Geometry: final body of the model. Coordinates: model frame, mm. A direction names the side the tool comes from. Round coordinates to 2 decimals unless told otherwise and drop trailing zeros. Loops run counter-clockwise (first coordinate to the right, second up) from the corner with the lowest first, then second, coordinate; pieces in that order, holes last. Notation, with made-up numbers: (41.5, -12) - (48.5, -12) arc R12 cw to (48.5, 8) - close; hole circle Ø3 at (73, 69). An arc over 180 degrees is marked (long way). Return JSON: item names as keys, results as strings. Group by question number.
1. Section C-C on z = 2. Return loops of the section in (x, y).
2. Section A-A on x = 0. Return loops of the section in (y, z) (1 decimal).
3. Section D-D on y = -15.5. Count the separate pieces of the cut face and the enclosed holes in it, and give its area (3 significant figures).
4. Draft query along X for faces 1 (the face through (39, 0, 4)), 2 (the face through (67.6, -12.5, 4.3)). Return one class per face: +X half, -X half, draft (parallel to the pull), parting line (faces both ways), or undercut.
5. Set-up query: faces 3 (the face through (16, 0, 4.762)), 4 (the face through (-13, 25.4, 7)), 5 (the face through (-16, -13, -4.762)). Return all of +Z, -Z, +X, -X, +Y, -Y with unobstructed straight access to the full face (end or side cutting, diameter ignored); none if empty.
6. Material intervals for probe 1 along X at (y, z) = (-19, -12); probe 2 along Y at (x, z) = (67.5, -10); probe 3 along X at (y, z) = (-13, -2), sorted ascending.
7. First-contact query: pin 1 Ø1 at (x, y) = (1.5, -18.5) entering from -Z; pin 2 Ø1.7 at (x, y) = (-16, -14) entering from +Z; pin 3 Ø3 at (x, z) = (-15, 1.5) entering from -Y; pin 4 Ø12 at (x, z) = (3, -4) entering from -Y. Flat tips, straight axial feed; report the tip coordinate or a pass-through.
from build123d import *

# Parameters (mm, degrees)
F0_R     = 14.2875
F1_DEPTH = 25.4
F2_DEPTH = 25.4


with BuildPart() as f1:
    # F0 (on Front) → F1 (new body)
    with BuildSketch(Plane.XZ):
        with BuildLine():
            ThreePointArc((5.9827839062, -27.9416699882), (22.2203586281, -17.9662541294), (28.575, 0))
            ThreePointArc((28.575, 0), (22.1191753976, 18.0906800516), (5.6687739472, 28.0070638757))
            ThreePointArc((5.6687739472, 28.0070638757), (-28.5745499588, -0.160373482), (5.9827839062, -27.9416699882))
        make_face()
        with BuildLine():
            ThreePointArc((-13.4703841816, 4.7625), (0, 14.2875), (13.4703841816, 4.7625))
            Line((13.4703841816, 4.7625), (19.05, 4.7625))
            Line((19.05, 4.7625), (19.05, -4.7625))
            Line((19.05, -4.7625), (13.4703841816, -4.7625))
            ThreePointArc((13.4703841816, -4.7625), (0, -14.2875), (-13.4703841816, -4.7625))
            Line((-13.4703841816, -4.7625), (-19.05, -4.7625))
            Line((-19.05, -4.7625), (-19.05, 4.7625))
            Line((-19.05, 4.7625), (-13.4703841816, 4.7625))
        make_face(mode=Mode.SUBTRACT)
        with BuildLine():
            ThreePointArc((5.6687739472, 28.0070638757), (22.1191753976, 18.0906800516), (28.575, 0))
            ThreePointArc((28.575, 0), (22.2203586281, -17.9662541294), (5.9827839062, -27.9416699882))
            Line((5.9827839062, -27.9416699882), (49.7382261223, -18.5728901119))
            ThreePointArc((49.7382261223, -18.5728901119), (34.9365884326, 0.6643681139), (51.0432019838, 18.8230459913))
            Line((51.0432019838, 18.8230459913), (5.6687739472, 28.0070638757))
        make_face()
        with BuildLine():
            ThreePointArc((73.025, 0), (66.3655558348, 14.469852318), (51.0432019838, 18.8230459913))
            ThreePointArc((51.0432019838, 18.8230459913), (34.9365884326, 0.6643681139), (49.7382261223, -18.5728901119))
            ThreePointArc((49.7382261223, -18.5728901119), (65.8533828367, -14.8931702866), (73.025, 0))
        make_face()
        with Locations((53.975, 0)):
            Circle(F0_R, mode=Mode.SUBTRACT)
    extrude(amount=F1_DEPTH)

    # F0 (on Front) → F2 (join)
    with BuildSketch(Plane.XZ):
        with BuildLine():
            ThreePointArc((5.9827839062, -27.9416699882), (22.2203586281, -17.9662541294), (28.575, 0))
            ThreePointArc((28.575, 0), (22.1191753976, 18.0906800516), (5.6687739472, 28.0070638757))
            ThreePointArc((5.6687739472, 28.0070638757), (-28.5745499588, -0.160373482), (5.9827839062, -27.9416699882))
        make_face()
        with BuildLine():
            ThreePointArc((-13.4703841816, 4.7625), (0, 14.2875), (13.4703841816, 4.7625))
            Line((13.4703841816, 4.7625), (19.05, 4.7625))
            Line((19.05, 4.7625), (19.05, -4.7625))
            Line((19.05, -4.7625), (13.4703841816, -4.7625))
            ThreePointArc((13.4703841816, -4.7625), (0, -14.2875), (-13.4703841816, -4.7625))
            Line((-13.4703841816, -4.7625), (-19.05, -4.7625))
            Line((-19.05, -4.7625), (-19.05, 4.7625))
            Line((-19.05, 4.7625), (-13.4703841816, 4.7625))
        make_face(mode=Mode.SUBTRACT)
        with BuildLine():
            ThreePointArc((-13.4703841816, -4.7625), (-14.2875, 0), (-13.4703841816, 4.7625))
            Line((-13.4703841816, 4.7625), (-19.05, 4.7625))
            Line((-19.05, 4.7625), (-19.05, -4.7625))
            Line((-19.05, -4.7625), (-13.4703841816, -4.7625))
        make_face()
    extrude(amount=-F2_DEPTH)


solid = f1.part
Taken from the geometry:
{
 "1": {"outline": "(-28.5, -25.4) - (-19.05, -25.4) - (-19.05, 0) - (-14.15, 0) - (-14.15, 25.4) - (-28.5, 25.4) - close; (19.05, -25.4) - (39.83, -25.4) - (39.83, 0) - (28.5, 0) - (28.5, 25.4) - (19.05, 25.4) - close; (68.12, -25.4) - (72.92, -25.4) - (72.92, 0) - (68.12, 0) - close"},
 "2": {"outline": "(-25.4, -28.6) - (25.4, -28.6) - (25.4, -14.3) - (-25.4, -14.3) - close; (-25.4, 14.3) - (25.4, 14.3) - (25.4, 28.6) - (-25.4, 28.6) - close"},
 "3": {"separate pieces": "1", "enclosed holes": "2", "area": "3,020 mm2"},
 "4": {"face 1": "draft", "face 2": "undercut"},
 "5": {"face 3": "+Y, -Y", "face 4": "+Z, -Z, +X, -X, +Y", "face 5": "-Y"},
 "6": {"probe 1": "-25.93 to -7.75, 7.75 to 46.22, 61.73 to 68.77", "probe 2": "-25.4 to 0", "probe 3": "-28.5 to -19.05, 19.05 to 39.83, 68.12 to 72.92"},
 "7": {"pin 1": "z = -28.56", "pin 2": "z = 24.23", "pin 3": "y = 0", "pin 4": "through"}
}
